Here's how the part is built. I have some questions about the finished solid (model axes, mm). A direction names the side the tool comes from. Coordinates: 2 decimals unless noted, no trailing zeros. Loops run counter-clockwise (first coordinate to the right, second up) from the corner with the lowest first, then second, coordinate; pieces in that order, holes last. Notation, with made-up numbers: M -7,-24.75 L 14,-24.75 A8 cw 14,-14.75 Z; hole C 5,1 d6. An arc over 180 degrees is marked long. Use CSV: the item, a comma, the result in double quotes. Start each with the question number.
Q1. If we section it at C-C (y = 34.5): Please give me the cut outline in (x, z).
Q2. Which directions (+Z, -Z, +X, -X, +Y, -Y) give clear straight access to the entire face, cutting with the end or side of a thin tool? Please do faces 1 (the flat face through (-6, 33, -1)), 2 (the flat face through (-6, 33, -11)), 3 (the flat face through (2.5, -10, -6)), 4 (the flat face through (-3, 20, -6)).
Q3. If we section it at B-B (x = -6.75): Please give me the cut outline in (y, z).
Q4. If we mould it in two halves opening along Y, with no side actions, what happens to faces 5 (the flat face through (-6, 29, -1)), 6 (the flat face through (-14.5, -10, -6)), 7 (the flat face through (-6, 39, -6)), 8 (the flat face through (-6, 10, -12))? For each: +Y half, -Y half, draft (parallel to the pull), parting line (faces both ways), or undercut.
Q5. If we section it at D-D (x = -1): Please give me the cut outline in (y, z).
Q6. If we section it at A-A (z = -2.75): Please give me the cut outline in (x, y).
Q7. For pin 1 Ø2 at (x, z) = (-5.5, -0.5) entering from +Y; pin 2 Ø13 at (y, z) = (34, -5.5) entering from +X; pin 3 Ø6 at (y, z) = (-9.5, 1) entering from -X, each with a flat end and sliding along its axis, tell me the tip position at first contact or that it passes through.
Q8. Please list where these lines run through material, in increasing order: probe 1 along Y at (x, z) = (-5, -11.75); probe 2 along Y at (x, z) = (-6.75, 0.5); probe 3 along Z at (x, y) = (-8, -13). Write a range as [from, to].
Autodesk Inventor part; units mm, degrees
ref_plane "YZ Plane" through (0, 0, 0) normal (1, 0, 0) x (0, 1, 0)
ref_plane "XZ Plane" through (0, 0, 0) normal (0, 1, 0) x (-1, 0, 0)
ref_plane "XY Plane" through (0, 0, 0) normal (0, 0, 1) x (1, 0, 0)
sketch "Sketch1" plane through (0, 0, 0) normal (0, 1, 0) x (-1, 0, 0)
  line L0 (0, 0) -> (12, 0)
  line L1 (12, 0) -> (12, -12)
  line L2 (12, -12) -> (0, -12)
  line L3 (0, -12) -> (0, 0)
  dimension "d0" = 12
  dimension "d1" = 12
extrude "Extrusion1" add sketch "Sketch1" along normal blind 20
ref_plane "Work Plane1" through (-6, 0, 0) normal (1, 0, 0) x (0, 0, -1)
sketch "Sketch2" plane through (-6, 0, 0) normal (1, 0, 0) x (0, 0, -1)
  line L0 (0, 20) -> (12, 20)
  line L1 (6, 20) -> (4, 20)
  line L2 (12, 20) -> (0, 20)
  line L3 (4, 20) -> (4, 29)
  line L4 (4, 29) -> (-2, 29)
  line L5 (-2, 29) -> (-2, 33)
  line L6 (-2, 33) -> (4, 33)
  line L7 (4, 33) -> (4, 39)
  line L8 (4, 39) -> (8, 39)
  line L9 (8, 39) -> (8, 33)
  line L10 (8, 33) -> (14, 33)
  line L11 (14, 33) -> (14, 29)
  line L12 (14, 29) -> (3, 29)
  line L13 (3, 29) -> (3, 20)
  line L14 (8, 29) -> (8, 20)
  line L15 (6, 20) -> (8, 20)
  point P0 (0, 0)
  dimension "d4" = 2
  dimension "d5" = 9
  dimension "d6" = 6
  dimension "d7" = 4
  dimension "d8" = 6
  dimension "d9" = 4
  dimension "d10" = 6
extrude "Extrusion2" add sketch "Sketch2" along normal mid plane 4 contours L3 L12 L14 L0 | L4 L5 L6 L7 L8 L9 L10 L11 L12
sketch "Sketch3" plane through (0, 0, 0) normal (0, -1, 0) x (1, 0, 0)
  line L0 (-12, 0) -> (0, 0)
  line L1 (0, 0) -> (0, -12)
  line L2 (0, 0) -> (2.5, 0)
  line L3 (2.5, 0) -> (2.5, 2.5)
  line L4 (2.5, 2.5) -> (-14.5, 2.5)
  line L5 (-14.5, 2.5) -> (-14.5, -14.5)
  line L6 (-14.5, -14.5) -> (2.5, -14.5)
  line L7 (2.5, -14.5) -> (2.5, 2.5)
  dimension "d15" = 2.5
  dimension "d16" = 2.5
  dimension "d17" = 17
  dimension "d18" = 17
extrude "Extrusion3" add sketch "Sketch3" along normal blind 20
sketch "Sketch4" plane through (0, -20, 0) normal (0, -1, 0) x (1, 0, 0)
  line L0 (2.5, -14.5) -> (2.5, 2.5)
  line L1 (2.5, 2.5) -> (2.5, 5)
  line L2 (2.5, 5) -> (5, 5)
  line L3 (5, 5) -> (-17, 5)
  line L4 (-17, 5) -> (-17, -17)
  line L5 (-17, -17) -> (5, -17)
  line L6 (5, -17) -> (5, 5)
  point P0 (0, 0)
  dimension "d21" = 2.5
  dimension "d22" = 2.5
  dimension "d23" = 22
  dimension "d24" = 22
extrude "Extrusion4" add sketch "Sketch4" along normal blind 20
properties part number "tiered-king"
Results below:
1,outline,"M -8,-8 L -4,-8 L -4,-4 L -8,-4 Z"
2,face 1,"+Z, +X, -X, +Y"
2,face 2,"-Z, +X, -X, +Y"
2,face 3,"+Z, -Z, +X, +Y"
2,face 4,"none"
3,outline,"M -40,-17 L -20,-17 L -20,-14.5 L 0,-14.5 L 0,-12 L 20,-12 L 20,-8 L 29,-8 L 29,-14 L 33,-14 L 33,-8 L 39,-8 L 39,-4 L 33,-4 L 33,2 L 29,2 L 29,-4 L 20,-4 L 20,0 L 0,0 L 0,2.5 L -20,2.5 L -20,5 L -40,5 Z"
4,face 5,"undercut"
4,face 6,"draft"
4,face 7,"+Y half"
4,face 8,"undercut"
5,outline,"M -40,-17 L -20,-17 L -20,-14.5 L 0,-14.5 L 0,-12 L 20,-12 L 20,0 L 0,0 L 0,2.5 L -20,2.5 L -20,5 L -40,5 Z"
6,outline,"M -17,-40 L 5,-40 L 5,-20 L 2.5,-20 L 2.5,0 L 0,0 L 0,20 L -12,20 L -12,0 L -14.5,0 L -14.5,-20 L -17,-20 Z; M -8,29 L -4,29 L -4,33 L -8,33 Z"
7,pin 1,"y = 33"
7,pin 2,"x = -4"
7,pin 3,"x = -14.5"
8,probe 1,"[-40, 20], [29, 33]"
8,probe 2,"[-40, 0], [29, 33]"
8,probe 3,"[-14.5, 2.5]"
